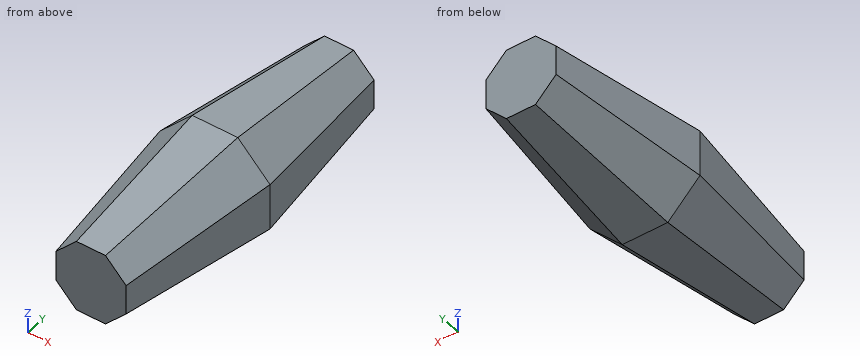
from build123d import *

# Parameters (mm, degrees)
BOSS_EXTRUDE1_DEPTH = 50
BOSS_EXTRUDE1_DRAFT = -7
MIRROR1_DEPTH       = 50
MIRROR1_DRAFT       = 7


# Read off the part's stored shape, not the designer's step: Mirror1
with BuildPart() as part:
    # Sketch2 → Boss-Extrude1 (with draft: the straight prism first)
    with BuildSketch(Plane(origin=(0, 0, 0), x_dir=(1, 0, 0), z_dir=(0, 1, 0))):
        Polygon((-10.863961031, 4.5), (-10.863961031, -4.5), (-4.5, -10.863961031), (4.5, -10.863961031), (10.863961031, -4.5), (10.863961031, 4.5), (4.5, 10.863961031), (-4.5, 10.863961031), align=None)
    extrude(amount=BOSS_EXTRUDE1_DEPTH)
    # Boss-Extrude1: the draft: its side faces are tilted about the plane it starts from
    boss_extrude1_sides = [part.faces().sort_by_distance(p)[0] for p in [
        (-10.863961031, 25, 0),
        (-7.681980515, 25, 7.681980515),
        (0, 25, 10.863961031),
        (7.681980515, 25, 7.681980515),
        (10.863961031, 25, 0),
        (7.681980515, 25, -7.681980515),
        (0, 25, -10.863961031),
        (-7.681980515, 25, -7.681980515),
    ]]
    draft(boss_extrude1_sides, Plane(origin=(0, 0, 0), x_dir=(1, 0, 0), z_dir=(0, 1, 0)), BOSS_EXTRUDE1_DRAFT)


with BuildPart() as mirror1_tool:
    # Mirror1 outline → Mirror1 (with draft: the straight prism first)
    with BuildSketch(Plane(origin=(0, 100, 0), x_dir=(1, 0, 0), z_dir=(0, 1, 0))):
        Polygon((-10.863961031, -4.5), (-4.5, -10.863961031), (4.5, -10.863961031), (10.863961031, -4.5), (10.863961031, 4.5), (4.5, 10.863961031), (-4.5, 10.863961031), (-10.863961031, 4.5), align=None)
    extrude(amount=-MIRROR1_DEPTH)
    # Mirror1: the draft: its side faces are tilted about the plane it starts from
    mirror1_sides = [mirror1_tool.faces().sort_by_distance(p)[0] for p in [
        (-7.681980515, 75, 7.681980516),
        (0, 75, 10.863961031),
        (7.681980516, 75, 7.681980515),
        (10.863961031, 75, 0),
        (7.681980515, 75, -7.681980516),
        (0, 75, -10.863961031),
        (-7.681980516, 75, -7.681980515),
        (-10.863961031, 75, 0),
    ]]
    draft(mirror1_sides, Plane(origin=(0, 100, 0), x_dir=(1, 0, 0), z_dir=(0, 1, 0)), MIRROR1_DRAFT)


with BuildPart() as part_1:
    add(part.part)

    # Mirror1: add mirror1_tool
    add(mirror1_tool.part)


solid = part_1.part
Read the model definition and answer for the solid it produces. Units are mm, in the model's axes. Coordinates: 2 decimals unless noted, no trailing zeros. Write each loop counter-clockwise with the first axis right and the second up, starting at its lowest first coordinate (ties: lowest second). Pieces come first, ordered by that corner, then holes. Notation, with made-up numbers: (25, 67.25) - (75, 67.25) arc R23 cw to (75, 79.25) - close; hole circle Ø9 at (41, 67.25). An arc over 180 degrees is marked (long way). One line per question, with ' | ' between items.
Q1. Find section B-B, the plane x = 2. Write down the section's boundary in (y, z).
Result set:
outline: (0, -10.86) - (50, -17) - (100, -10.86) - (100, 10.86) - (50, 17) - (0, 10.86) - close
Q2. Each of these flat-tipped pins is pushed along its axis until it touches: P1, Ø10, axis at y = 73.5, z = -12, coming from the +X side; P2, Ø5, axis at x = 4, y = 16.5, coming from the -Z side; P3, Ø1, axis at y = 45.5, z = 1.5, coming from the -X side. Where does it stop, or does it pass through?
Result set:
P1: x = 13.04 | P2: z = -13.2 | P3: x = -16.51
Q3. Consider L1, parallel to Z at x = -8.5, y = 10.5; L2, parallel to X at y = 58, z = -2.5; L3, parallel to X at y = 74.5, z = -3.5. Determine where each line is inside the solid, lowest interval first. Write a range as [from, to].
Result set:
L1: [-8.69, 8.69] | L2: [-16.02, 16.02] | L3: [-13.99, 13.99]
Q4. Find section D-D, the plane y = 10. Write down the section's boundary in (x, z).
Result set:
outline: (-12.09, -5.01) - (-5.01, -12.09) - (5.01, -12.09) - (12.09, -5.01) - (12.09, 5.01) - (5.01, 12.09) - (-5.01, 12.09) - (-12.09, 5.01) - close
Q5. Find section C-C, the plane z = 8. Write down the section's boundary in (x, y), plus the area to 3 significant figures.
Result set:
outline: (-16.05, 50) - (-7.36, 0) - (7.36, 0) - (16.05, 50) - (7.36, 100) - (-7.36, 100) - close | area: 2,340 mm^2
Q6. Find section A-A, the plane y = 53. Write down the section's boundary in (x, z), plus the area to 3 significant figures.
Result set:
outline: (-16.63, -6.89) - (-6.89, -16.63) - (6.89, -16.63) - (16.63, -6.89) - (16.63, 6.89) - (6.89, 16.63) - (-6.89, 16.63) - (-16.63, 6.89) - close | area: 917 mm^2
